Input: dimensioned drawing with shaded views. Units: mm. Origin: part minimum x, y, z. A direction names the side the tool comes from. Give positions to 0.01 mm unless a question says otherwise; leave off trailing zeros. Write each loop counter-clockwise with the first axis right and the second up, starting at its lowest first coordinate (ties: lowest second). Pieces come first, ordered by that corner, then holes.
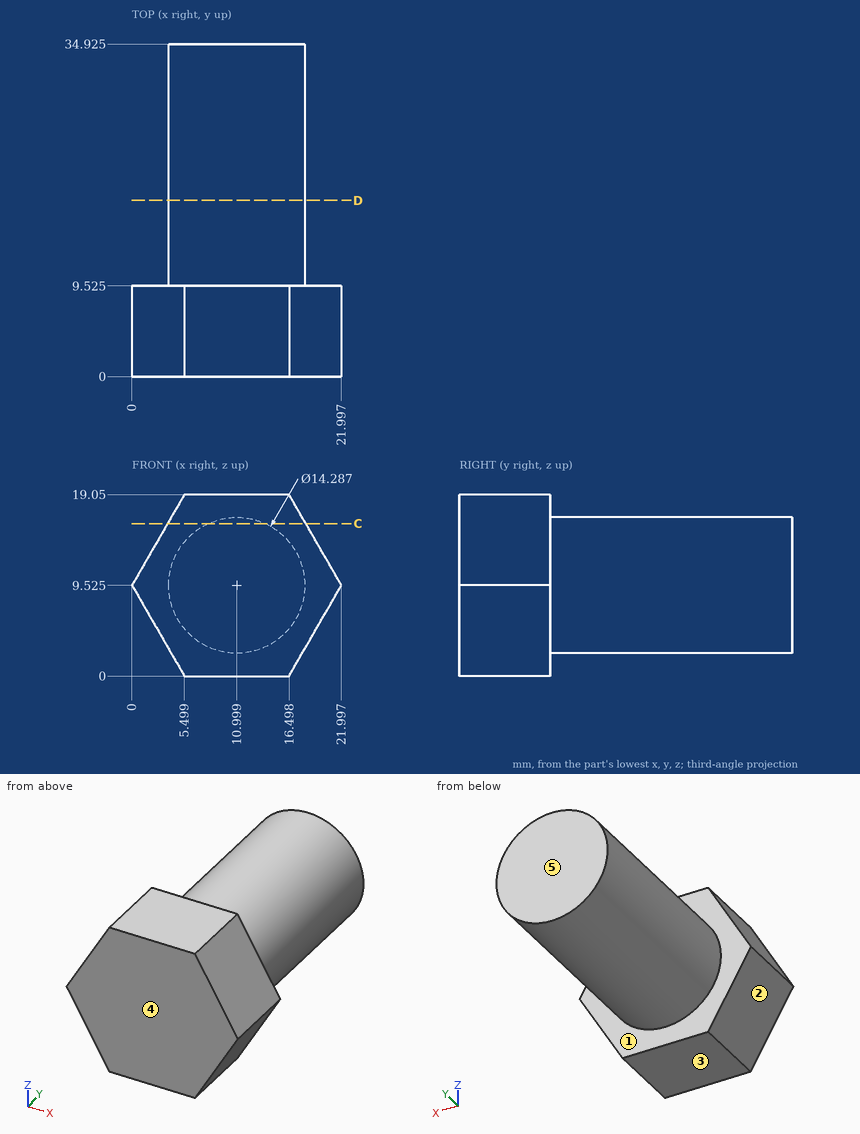
Item 1: Section D-D, the plane y = 18.5. Return the cut outline in (x, z) (1 decimal).
Found:
outline: circle Ø14.3 at (11, 9.5)
Item 2: Pin query (flat end, axial travel): pin 1 Ø8 at (x, z) = (8, 11.5) entering from -Y; pin 2 Ø10 at (y, z) = (20.5, 4.5) entering from -X (1 decimal); pin 3 Ø6 at (x, y) = (9, 23.5) entering from -Z. Return the tip coordinate at first contact, or that it passes through.
Found:
pin 1: stops at y = 0
pin 2: stops at x = 3.9
pin 3: stops at z = 2.38
Item 3: Section C-C, the plane z = 16. Return the cut outline in (x, y) (1 decimal), plus the area to 3 significant figures.
Found:
outline: (3.7, 0) - (18.3, 0) - (18.3, 9.5) - (14, 9.5) - (14, 34.9) - (8, 34.9) - (8, 9.5) - (3.7, 9.5) - close
area: 292 mm2
Item 4: Pull-direction query (Y, two-part tool) for the marked faces 3, 4 and 5; classes: +Y half, -Y half, draft (parallel to the pull), parting line (faces both ways), or undercut.
Found:
face 3: draft
face 4: -Y half
face 5: +Y half
Item 5: Line query: L1, parallel to Y at x = 14.5, z = 16.75 (1 decimal); L2, parallel to Z at x = 11.25, y = 25 (1 decimal); L3, parallel to X at y = 17.5, z = 3.75 (1 decimal). Output: solid intervals per line, ascending.
Found:
L1: y = 0 to 9.5
L2: z = 2.4 to 16.7
L3: x = 6.8 to 15.2
Item 6: Reachability of the marked faces 1 and 2 from +Z, -Z, +X, -X, +Y, -Y: full face, straight path, thin tool, end or side. Return the list, or none.
Found:
face 1: +Y
face 2: -Z, -X, +Y, -Y
